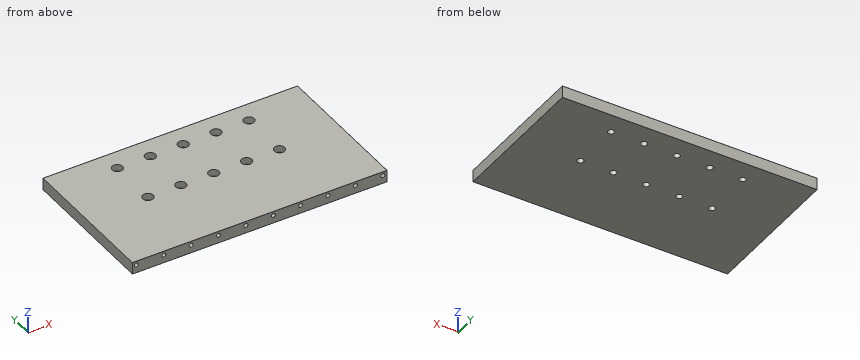
```python
from build123d import *

# Parameters (mm, degrees)
SKETCH2_W            = 635
SKETCH2_H            = 360
BOSS_EXTRUDE1_DEPTH  = 30
SKETCH3_R            = 13
CUT_EXTRUDE2_DEPTH   = 17
SKETCH4_R            = 8
CUT_EXTRUDE3_DEPTH   = 14
LPATTERN1_COUNT      = 5
LPATTERN1_PITCH      = 82
LPATTERN1_COUNT_DIR2 = 2
LPATTERN1_PITCH_DIR2 = 123
FILLET1_R            = 0.3
SKETCH7_R            = 5
CUT_EXTRUDE4_DEPTH   = 18
LPATTERN2_COUNT      = 10
LPATTERN2_PITCH      = 68.3


with BuildPart() as part:
    # Sketch2 → Boss-Extrude1 (new body)
    with BuildSketch(Plane.XY):
        with Locations((317.5, 180)):
            Rectangle(SKETCH2_W, SKETCH2_H)
    extrude(amount=BOSS_EXTRUDE1_DEPTH)

    # Sketch3 → Cut-Extrude2 (cut)
    with BuildSketch(Plane.XY.offset(30)):
        with Locations((153.5, 308)):
            Circle(SKETCH3_R)
    cut_extrude2 = extrude(amount=-CUT_EXTRUDE2_DEPTH, mode=Mode.SUBTRACT)

    # Sketch4 → Cut-Extrude3 (cut, through all)
    with BuildSketch(Plane.XY.offset(13)):
        with Locations((153.5, 308)):
            Circle(SKETCH4_R)
    cut_extrude3 = extrude(amount=-CUT_EXTRUDE3_DEPTH, mode=Mode.SUBTRACT)

    # LPattern1: Cut-Extrude2, Cut-Extrude3 5 × 2
    with Locations(*[(i * LPATTERN1_PITCH, -j * LPATTERN1_PITCH_DIR2, 0) for i in range(LPATTERN1_COUNT) for j in range(LPATTERN1_COUNT_DIR2) if (i, j) != (0, 0)]):
        add(cut_extrude2, mode=Mode.SUBTRACT)
        add(cut_extrude3, mode=Mode.SUBTRACT)

    # Fillet1
    fillet1_edges = [part.edges().sort_by_distance(p)[0] for p in [
        (635, 180, 30),
        (317.5, 360, 30),
        (317.5, 360, 0),
        (635, 180, 0),
        (317.5, 0, 0),
        (0, 180, 0),
        (0, 360, 15),
        (635, 360, 15),
        (635, 0, 15),
        (0, 0, 15),
        (317.5, 0, 30),
    ]]
    fillet(fillet1_edges, radius=FILLET1_R)

    # Sketch7 → Cut-Extrude4 (cut)
    with BuildSketch(Plane.XZ):
        with Locations((10, 20)):
            Circle(SKETCH7_R)
    cut_extrude4 = extrude(amount=-CUT_EXTRUDE4_DEPTH, mode=Mode.SUBTRACT)

    # LPattern2: Cut-Extrude4 ×10
    with Locations(*[(i * LPATTERN2_PITCH, 0, 0) for i in range(1, LPATTERN2_COUNT)]):
        add(cut_extrude4, mode=Mode.SUBTRACT)


solid = part.part
```
Input: part model. Units: mm. Frame: model coordinates. Give positions to 0.01 mm unless a question says otherwise; leave off trailing zeros. Order: outer loops, then holes, each group sorted by start corner. A loop starts at its lowest first (then second) coordinate and runs counter-clockwise, first axis right, second up.
1. Section B-B on z = 20. Give the number of separate pieces and of enclosed holes in the cut face, and give its area (3 significant figures).
Derived:
separate pieces: 1
enclosed holes: 10
area: 221,000 mm2
2. Material intervals for L1, parallel to Y at x = 154.5, z = 24.5; L2, parallel to Z at x = 351.5, y = 8.25; L3, parallel to Y at x = 486, z = 23.5, sorted ascending.
Derived:
L1: y = 0 to 172.04, 197.96 to 295.04, 320.96 to 360
L2: z = 0 to 15, 25 to 30
L3: y = 18 to 172.8, 197.2 to 295.8, 320.2 to 360
3. Section A-A on x = 235.5. Return the cut outline in (y, z), and give its area (3 significant figures).
Derived:
outline: (0, 0.3) arc R0.3 ccw to (0.3, 0) - (177, 0) - (177, 13) - (172, 13) - (172, 30) - (0.3, 30) arc R0.3 ccw to (0, 29.7) - close; (193, 0) - (300, 0) - (300, 13) - (295, 13) - (295, 30) - (198, 30) - (198, 13) - (193, 13) - close; (316, 0) - (359.7, 0) arc R0.3 ccw to (360, 0.3) - (360, 29.7) arc R0.3 ccw to (359.7, 30) - (321, 30) - (321, 13) - (316, 13) - close
area: 9,500 mm2
4. Pin query (flat end, axial travel): pin 1 (6 mm diameter, centred on x = 556.4, z = 20, fed in from -Y); pin 2 (8 mm diameter, centred on x = 230.5, y = 307, fed in from +Z); pin 3 (23.5 mm diameter, centred on x = 399.5, y = 308, fed in from -Z). Return the tip coordinate at first contact, or that it passes through.
Derived:
pin 1: stops at y = 18
pin 2: stops at z = 13
pin 3: stops at z = 0
